Input: part model. Units: mm. Frame: model coordinates. Coordinates: 2 decimals unless noted, no trailing zeros. Write each loop counter-clockwise with the first axis right and the second up, starting at its lowest first coordinate (ties: lowest second). Pieces come first, ordered by that corner, then holes. Notation, with made-up numbers: M -25.75,15 L -11.75,15 A21 ccw -11.75,38 Z; hole C 0,-10.5 d5. An arc over 180 degrees is marked long. Use one line per item in the form item = value.
from build123d import *

# Parameters (mm, degrees)
SKETCH1_W            = 6.4
SKETCH1_H            = 6.4
BOSS_EXTRUDE1_DEPTH  = 1
M3_CLEARANCE_HOLE1_D = 3.2
FILLET1_R            = 0.3


with BuildPart() as part:
    # Sketch1 → Boss-Extrude1 (new body)
    with BuildSketch(Plane(origin=(0, 0, 0), x_dir=(1, 0, 0), z_dir=(0, 1, 0))):
        Rectangle(SKETCH1_W, SKETCH1_H)
    extrude(amount=BOSS_EXTRUDE1_DEPTH)

    # M3 Clearance Hole1 (through all)
    with Locations(Plane(origin=(0, 1, 0), x_dir=(1, 0, 0), z_dir=(0, 1, 0))):
        with Locations((0, 0)):
            Hole(M3_CLEARANCE_HOLE1_D / 2)

    # Fillet1
    fillet1_edges = [part.edges().sort_by_distance(p)[0] for p in [
        (3.2, 0.5, 3.2),
        (3.2, 0.5, -3.2),
        (-3.2, 0.5, -3.2),
        (-3.2, 0.5, 3.2),
    ]]
    fillet(fillet1_edges, radius=FILLET1_R)


solid = part.part
(1) Line query: probe 1 along Z at (x, y) = (0, 0.45); probe 2 along X at (y, z) = (0.2, -0.5); probe 3 along X at (y, z) = (0.25, -1). Output: solid intervals per line, ascending.
Computed:
probe_1 = -3.2 to -1.6, 1.6 to 3.2
probe_2 = -3.2 to -1.52, 1.52 to 3.2
probe_3 = -3.2 to -1.25, 1.25 to 3.2
(2) Section query B-B on x = 0. Return the cut outline in (y, z).
Computed:
outline = M 0,-3.2 L 1,-3.2 L 1,-1.6 L 0,-1.6 Z; M 0,1.6 L 1,1.6 L 1,3.2 L 0,3.2 Z
(3) Section query A-A on z = 0. Return the cut outline in (x, y).
Computed:
outline = M -3.2,0 L -1.6,0 L -1.6,1 L -3.2,1 Z; M 1.6,0 L 3.2,0 L 3.2,1 L 1.6,1 Z
(4) Pull-direction query (Z, two-part tool) for faces 1 (the flat face through (0, 0.5, 3.2)), 2 (the flat face through (0, 0.5, -3.2)), 3 (the cylindrical face through (1.27, 0.49, 0.97)), 4 (the flat face through (-1.5, 1, -1.5)); classes: pulls with the +Z half, pulls with the -Z half, needs draft (parallel to the pull), parting line crosses it, or undercut.
Computed:
face_1 = pulls with the +Z half
face_2 = pulls with the -Z half
face_3 = undercut
face_4 = needs draft
(5) Section query C-C on y = 0.4. Return the cut outline in (x, z).
Computed:
outline = M -3.2,-2.9 A0.3 ccw -2.9,-3.2 L 2.9,-3.2 A0.3 ccw 3.2,-2.9 L 3.2,2.9 A0.3 ccw 2.9,3.2 L -2.9,3.2 A0.3 ccw -3.2,2.9 Z; hole C 0,0 d3.2
